CAD build for the part. Positions are in the model's coordinates, mm. Face numbers are marked on the shaded views. A direction names the side the tool comes from. Round coordinates to 2 decimals unless told otherwise and drop trailing zeros. Loops run counter-clockwise (first coordinate to the right, second up) from the corner with the lowest first, then second, coordinate; pieces in that order, holes last. Notation, with made-up numbers: M 34,27 L 45,27 A20 cw 45,60 Z; hole C 7,-5 d6. An arc over 180 degrees is marked long. Put each result on its own line as item: value. Start each with the question number.
from build123d import *

# Parameters (mm, degrees)
F1_DEPTH = 10
F2_R     = 1.876476
F3_DEPTH = 6


with BuildPart() as f1:
    # F0 (on Top) → F1 (new body)
    with BuildSketch(Plane.XY):
        with BuildLine():
            ThreePointArc((17.866252, 11.169709), (0, 26.979497), (-17.866252, 11.169709))
            Line((-17.866252, 11.169709), (-17.866252, 6))
            Line((-17.866252, 6), (-30, 6))
            Line((-30, 6), (-30, 0))
            Line((-30, 0), (-11.670343, 0))
            Line((-11.670343, 0), (-11.670343, 5.692855))
            ThreePointArc((-11.670343, 5.692855), (0, 20.486258), (11.670343, 5.692855))
            Line((11.670343, 5.692855), (11.670343, 0))
            Line((11.670343, 0), (30, 0))
            Line((30, 0), (30, 6))
            Line((30, 6), (17.866252, 6))
            Line((17.866252, 6), (17.866252, 11.169709))
        make_face()
    extrude(amount=F1_DEPTH)

    # F2 (on Front) → F3 (cut)
    with BuildSketch(Plane.XZ):
        with Locations((-20.210268, 4.529888)):
            Circle(F2_R)
        with Locations((20.210268, 4.529888)):
            Circle(F2_R)
    extrude(amount=-F3_DEPTH, mode=Mode.SUBTRACT)


solid = f1.part
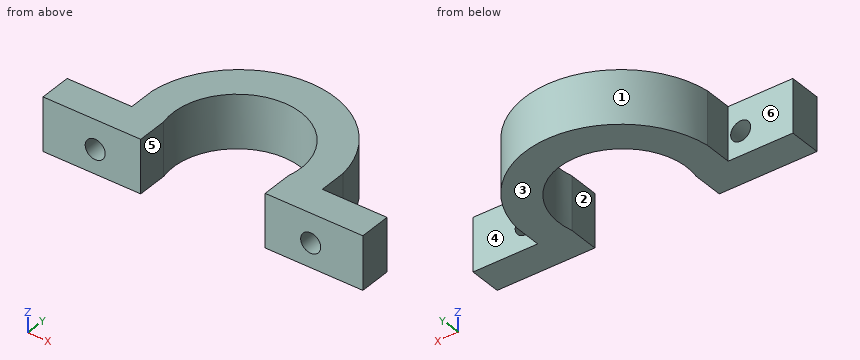
(1) Drill centre lines: line 1 along X through (y, z) = (5.5, 4); line 2 along X through (y, z) = (4, 9.25); line 3 along X through (y, z) = (1.75, 3.25). Where is each one in solid material? Low to high.
(2) Mould opens along X. For the marked faces 1, 2 and 3 say: +X half, -X half, draft (parallel to the pull), parting line (faces both ways), or undercut.
(3) Cut at D-D on x = 0. List the corners of the cut face in (y, z).
(4) Cut at B-B on z = 5.75. List the corners of the cut face in (x, y).
(5) Flat gauge pins, fed straight in: pin 1 Ø1.5 at (y, z) = (10, 7) entering from -X; pin 2 Ø1.5 at (y, z) = (16.5, 6.5) entering from -X; pin 3 Ø12 at (x, y) = (18, 17.5) entering from -Z; pin 4 Ø1 at (x, z) = (20, 7) entering from +Y. Where does each tip first touch, or does it go through?
(6) Cut at C-C on z = 1. List the corners of the cut face in (x, y).
(7) Tool access for the marked faces 4, 5 and 6: list every direction of +Z, -Z, +X, -X, +Y, -Y with a clear straight run to the whole face (end or side of a thin tool).
(8) Cut at A-A on y = 8.25. List the corners of the cut face in (x, z), and give its area (3 significant figures).
Taken from the geometry:
1. line 1: -30 to -22.01, -18.41 to -11.67, 11.67 to 18.41, 22.01 to 30
1. line 2: -30 to -11.67, 11.67 to 30
1. line 3: -30 to -21.58, -18.84 to -11.67, 11.67 to 18.84, 21.58 to 30
2. face 1: parting line
2. face 2: undercut
2. face 3: draft
3. outline: M 20.49,0 L 26.98,0 L 26.98,10 L 20.49,10 Z
4. outline: M -30,0 L -21.64,0 L -21.64,6 L -30,6 Z; M -18.78,0 L -11.67,0 L -11.67,5.69 A12 cw long 11.67,5.69 L 11.67,0 L 18.78,0 L 18.78,6 L 17.87,6 L 17.87,11.17 A18 ccw -17.87,11.17 L -17.87,6 L -18.78,6 Z; M 21.64,0 L 30,0 L 30,6 L 21.64,6 Z
5. pin 1: x = -17.87
5. pin 2: x = -16.68
5. pin 3: z = 0
5. pin 4: y = 6
6. outline: M -30,0 L -11.67,0 L -11.67,5.69 A12 cw long 11.67,5.69 L 11.67,0 L 30,0 L 30,6 L 17.87,6 L 17.87,11.17 A18 ccw -17.87,11.17 L -17.87,6 L -30,6 Z
7. face 4: +Z, -Z, +X, +Y
7. face 5: +Z, -Z, -Y
7. face 6: +Z, -Z, -X, +Y
8. outline: M -17.87,0 L -12,0 L -12,10 L -17.87,10 Z; M 12,0 L 17.87,0 L 17.87,10 L 12,10 Z
8. area: 117 mm2
